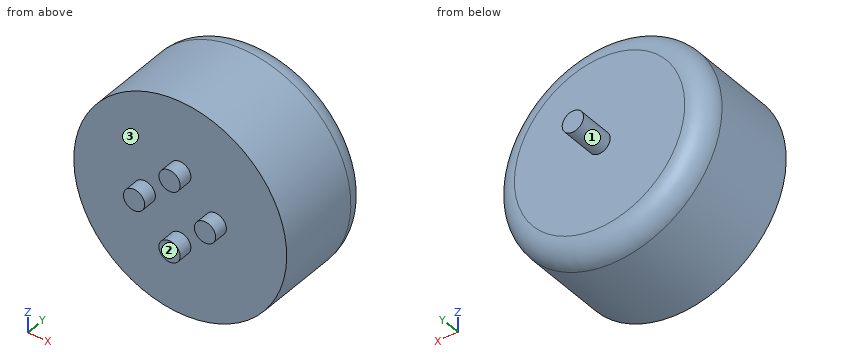
from build123d import *

# Parameters (mm, degrees)
SKETCH_2_R      = 15
EXTRUDE_1_DEPTH = 15
FILLET_1_R      = 3
SKETCH_3_R      = 1.5
EXTRUDE_2_DEPTH = 5
SKETCH_4_R      = 1.5
EXTRUDE_3_DEPTH = 2


with BuildPart() as part:
    # 草图2 → 凸台-拉伸1 (new body)
    with BuildSketch(Plane(origin=(0, 0, 0), x_dir=(1, 0, 0), z_dir=(0, 1, 0))):
        with Locations(Location((0, 0, 0), (0, 0, 270))):
            Circle(SKETCH_2_R)
    extrude(amount=EXTRUDE_1_DEPTH)

    # 圆角1
    fillet_1_edges = [part.edges().sort_by_distance(p)[0] for p in [
        (0, 15, -15),
    ]]
    fillet(fillet_1_edges, radius=FILLET_1_R)

    # 草图3 → 凸台-拉伸2 (add)
    with BuildSketch(Plane(origin=(0, 15, 0), x_dir=(1, 0, 0), z_dir=(0, 1, 0))):
        with Locations(Location((0, 0, 0), (0, 0, 270))):
            Circle(SKETCH_3_R)
    extrude(amount=EXTRUDE_2_DEPTH)

    # 草图4 → 凸台-拉伸3 (add)
    with BuildSketch(Plane.XZ):
        with Locations(Location((0, 5, 0), (0, 0, 90))):
            Circle(SKETCH_4_R)
        with Locations(Location((-5, 0, 0), (0, 0, 90))):
            Circle(SKETCH_4_R)
        with Locations(Location((5, 0, 0), (0, 0, 90))):
            Circle(SKETCH_4_R)
        with Locations(Location((0, -5, 0), (0, 0, 90))):
            Circle(SKETCH_4_R)
    extrude(amount=EXTRUDE_3_DEPTH)


solid = part.part
The listing builds one solid part. Answer for the finished solid, in the listing's coordinates (mm). Face numbers are marked on the shaded views. A direction names the side the tool comes from. Coordinates: 2 decimals unless noted, no trailing zeros. Loops run counter-clockwise (first coordinate to the right, second up) from the corner with the lowest first, then second, coordinate; pieces in that order, holes last.
1) Flat-ended cylindrical pins translate along their axes: pin 1 Ø1.5 at (x, z) = (-7.5, -9.5) entering from +Y; pin 2 Ø5 at (x, z) = (0.5, -11) entering from -Y; pin 3 Ø2 at (y, z) = (8.5, 7) entering from -X. Find the tip coordinate at first contact, or state that the pin passes through.
2) A tool of negligible diameter and unlimited length cuts with its end or side. For the marked faces 1, 2 and 3, from which of +Z, -Z, +X, -X, +Y, -Y can it reach the whole face along a straight path? Write none if from no direction.
3) Find the intervals of material crossed by L1, parallel to Y at x = -7.25, z = 3.5; L2, parallel to X at y = 5, z = -6.75; L3, parallel to Z at x = -11, y = 5.5, in increasing order.
4) Find section A-A on z = 0. Write down the section's boundary in (x, y), then the cut area to 3 significant figures.
5) Find section C-C on y = 17.5. Write down the section's boundary in (x, z), then the cut area to 3 significant figures.
6) Find section D-D on y = 4.25. Write down the section's boundary in (x, z), then the cut area to 3 significant figures.
7) Find section B-B on x = 0. Write down the section's boundary in (y, z).
Values:
1. pin 1: stops at y = 15
1. pin 2: stops at y = 0
1. pin 3: stops at x = -13.75
2. face 1: +Y
2. face 2: +Z, -Z, +X, -X, -Y
2. face 3: -Y
3. L1: y = 0 to 15
3. L2: x = -13.4 to 13.4
3. L3: z = -10.2 to 10.2
4. outline: (-15, 0) - (-6.5, 0) - (-6.5, -2) - (-3.5, -2) - (-3.5, 0) - (3.5, 0) - (3.5, -2) - (6.5, -2) - (6.5, 0) - (15, 0) - (15, 12) arc R3 ccw to (12, 15) - (1.5, 15) - (1.5, 20) - (-1.5, 20) - (-1.5, 15) - (-12, 15) arc R3 ccw to (-15, 12) - close
4. area: 473 mm2
5. outline: circle Ø3 at (0, 0)
5. area: 7.07 mm2
6. outline: circle Ø30 at (0, 0)
6. area: 707 mm2
7. outline: (-2, -6.5) - (0, -6.5) - (0, -15) - (12, -15) arc R3 ccw to (15, -12) - (15, -1.5) - (20, -1.5) - (20, 1.5) - (15, 1.5) - (15, 12) arc R3 ccw to (12, 15) - (0, 15) - (0, 6.5) - (-2, 6.5) - (-2, 3.5) - (0, 3.5) - (0, -3.5) - (-2, -3.5) - close
